from build123d import *

# Parameters (mm, degrees)
SKETCH_1_R      = 25
EXTRUDE_1_DEPTH = 1


with BuildPart() as part:
    # 草图1 → 凸台-拉伸1 (new body)
    with BuildSketch(Plane.XY):
        Circle(SKETCH_1_R)
        with BuildLine():
            Line((-1.6, 20.85), (-1.6, 18.430680942))
            ThreePointArc((-1.6, 18.430680942), (-7.079643499, 17.091771351), (-11.901088626, 14.163830326))
            Line((-11.901088626, 14.163830326), (-13.611805538, 15.874547238))
            ThreePointArc((-13.611805538, 15.874547238), (-15.874547238, 15.874547238), (-15.874547238, 13.611805538))
            Line((-15.874547238, 13.611805538), (-14.163830326, 11.901088626))
            ThreePointArc((-14.163830326, 11.901088626), (-17.091771351, 7.079643499), (-18.430680942, 1.6))
            Line((-18.430680942, 1.6), (-20.85, 1.6))
            ThreePointArc((-20.85, 1.6), (-22.45, 0), (-20.85, -1.6))
            Line((-20.85, -1.6), (-18.430680942, -1.6))
            ThreePointArc((-18.430680942, -1.6), (-17.091771351, -7.079643499), (-14.163830326, -11.901088626))
            Line((-14.163830326, -11.901088626), (-15.874547238, -13.611805538))
            ThreePointArc((-15.874547238, -13.611805538), (-15.874547238, -15.874547238), (-13.611805538, -15.874547238))
            Line((-13.611805538, -15.874547238), (-11.901088626, -14.163830326))
            ThreePointArc((-11.901088626, -14.163830326), (-7.079643499, -17.091771351), (-1.6, -18.430680942))
            Line((-1.6, -18.430680942), (-1.6, -20.85))
            ThreePointArc((-1.6, -20.85), (0, -22.45), (1.6, -20.85))
            Line((1.6, -20.85), (1.6, -18.430680942))
            ThreePointArc((1.6, -18.430680942), (7.079643499, -17.091771351), (11.901088626, -14.163830326))
            Line((11.901088626, -14.163830326), (13.611805538, -15.874547238))
            ThreePointArc((13.611805538, -15.874547238), (15.874547238, -15.874547238), (15.874547238, -13.611805538))
            Line((15.874547238, -13.611805538), (14.163830326, -11.901088626))
            ThreePointArc((14.163830326, -11.901088626), (17.091771351, -7.079643499), (18.430680942, -1.6))
            Line((18.430680942, -1.6), (20.85, -1.6))
            ThreePointArc((20.85, -1.6), (22.45, 0), (20.85, 1.6))
            Line((20.85, 1.6), (18.430680942, 1.6))
            ThreePointArc((18.430680942, 1.6), (17.091771351, 7.079643499), (14.163830326, 11.901088626))
            Line((14.163830326, 11.901088626), (15.874547238, 13.611805538))
            ThreePointArc((15.874547238, 13.611805538), (15.874547238, 15.874547238), (13.611805538, 15.874547238))
            Line((13.611805538, 15.874547238), (11.901088626, 14.163830326))
            ThreePointArc((11.901088626, 14.163830326), (7.079643499, 17.091771351), (1.6, 18.430680942))
            Line((1.6, 18.430680942), (1.6, 20.85))
            ThreePointArc((1.6, 20.85), (0, 22.45), (-1.6, 20.85))
        make_face(mode=Mode.SUBTRACT)
    extrude(amount=EXTRUDE_1_DEPTH)


solid = part.part
Read the model definition and answer for the solid it produces. Units are mm, in the model's axes. A direction names the side the tool comes from. Coordinates: 2 decimals unless noted, no trailing zeros. Loops run counter-clockwise (first coordinate to the right, second up) from the corner with the lowest first, then second, coordinate; pieces in that order, holes last. Notation, with made-up numbers: (72.25, -40) -> (101.25, -40) arc R26 ccw to (101.25, -11) -> close; hole circle Ø2 at (-5.5, 18). An arc over 180 degrees is marked (long way). Answer in a Markdown table with one row per item.
Item 1: A cutting plane is placed at A-A on x = -20. Determine the outline of the cut face in (y, z), plus the area to 3 significant figures.
Returned:
| item | result |
|---|---|
| outline | (-15, 0) -> (-1.6, 0) -> (-1.6, 1) -> (-15, 1) -> close; (1.6, 0) -> (15, 0) -> (15, 1) -> (1.6, 1) -> close |
| area | 26.8 mm^2 |
Item 2: For faces 4 (the flat face through (-2, 19, 0)), 5 (the cylindrical face through (-22.45, 0.04, 0.49)), determine the directions among +Z, -Z, +X, -X, +Y, -Y from which every point of the face is accessible in a straight line to the end or side of a thin tool.
Returned:
| item | result |
|---|---|
| face 4 | -Z, +X, -X, +Y, -Y |
| face 5 | +Z, -Z |
Item 3: Each of these flat-tipped pins is pushed along its axis until it touches: P1, Ø12, axis at x = 14, y = 19, coming from the -Z side; P2, Ø0.5, axis at x = -19, z = 0.5, coming from the +Y side; P3, Ø0.5, axis at y = 19, z = 0.5, coming from the +X side; P4, Ø0.5, axis at x = 20, z = 0.5, coming from the +Y side. Where does it stop, or does it pass through?
Returned:
| item | result |
|---|---|
| P1 | stops at z = 0 |
| P2 | stops at y = 16.54 |
| P3 | stops at x = 16.54 |
| P4 | stops at y = 15.33 |
Item 4: For a pull along Y with two mould halves and no side action, classify faces 1 (the cylindrical face through (23.846, 7.509, 0.493)), 2 (the flat face through (-2, 19, 1)), 3 (the cylindrical face through (17.12, 7.01, 0.49)) as released by +Y, released by -Y, zero draft, split by the parting line, or undercut.
Returned:
| item | result |
|---|---|
| face 1 | split by the parting line |
| face 2 | zero draft |
| face 3 | undercut |
Item 5: Straight lines are drawn through the part: line 1 along Y through (x, z) = (11, 0.75); line 2 along X through (y, z) = (17, 0.5); line 3 along X through (y, z) = (-13, 0.55). For each, find the intervals that lie inside material, in ascending order. Write a range as [from, to].
Returned:
| item | result |
|---|---|
| line 1 | y = [-22.45, -14.87], [14.87, 22.45] |
| line 2 | x = [-18.33, -7.3], [7.3, 18.33] |
| line 3 | x = [-21.35, -15.26], [15.26, 21.35] |
Item 6: A cutting plane is placed at C-C on y = 10.5. Determine the outline of the cut face in (x, z), plus the area to 3 significant figures.
Returned:
| item | result |
|---|---|
| outline | (-22.69, 0) -> (-15.23, 0) -> (-15.23, 1) -> (-22.69, 1) -> close; (15.23, 0) -> (22.69, 0) -> (22.69, 1) -> (15.23, 1) -> close |
| area | 14.9 mm^2 |
